Geometry check sheet. Reference: the model listing, model coordinates, mm. A direction names the side the tool comes from. Round coordinates to 2 decimals unless told otherwise and drop trailing zeros. Order: outer loops, then holes, each group sorted by start corner. A loop starts at its lowest first (then second) coordinate and runs counter-clockwise, first axis right, second up. Notation, with made-up numbers: (42.25, 18.5) - (55.25, 18.5) arc R6 ccw to (55.25, 25.5) - close; hole circle Ø10 at (68.5, 79.25). An arc over 180 degrees is marked (long way). One line per question, with ' | ' between items. Start each with the question number.
Q1. Material ranges on line 1 along Y through (x, z) = (11.5, -8); line 2 along Y through (x, z) = (5.25, 5.5); line 3 along X through (y, z) = (18.25, 2.75), recorded low to high.
Q2. Sectioned sample at B-B, the plane z = -6. Enter the section's corners in (x, y).
Q3. Tool access check on faces 1 (the face through (5, 15, 0)), 2 (the face through (17.465, 2.465, -0.14)). Record the directions out of +Z, -Z, +X, -X, +Y, -Y that give a thin tool (end or side, any length) a straight path to the whole face; none if there is none.
Q4. Sectioned sample at C-C, the plane y = 16.5. Enter the section's corners in (x, z).
Q5. Sectioned sample at D-D, the plane z = 0. Enter the section's corners in (x, y), then the cut area to 3 significant figures.
Q6. Gauge pin test, flat ends, axial feed: P1, Ø12, axis at x = 12, z = 3.5, coming from the +Y side; P2, Ø11, axis at x = 4.5, z = 2.5, coming from the +Y side; P3, Ø5, axis at y = 3, z = -3.5, coming from the -X side; P4, Ø4, axis at x = -3.5, y = 3, coming from the +Z side. Record the tip position at first contact, or that the pin passes through.
Q7. Sectioned sample at A-A, the plane x = 7. Enter the section's corners in (y, z), then the cut area to 3 significant figures.
```python
from build123d import *

# Parameters (mm, degrees)
EXTRUDE_2_DEPTH = 20
EXTRUDE_3_DEPTH = 15
EXTRUDE_4_DEPTH = 5


with BuildPart() as part:
    # Sketch 1 → Extrude 2 (new body)
    with BuildSketch(Plane(origin=(0, 0, 0), x_dir=(1, 0, 0), z_dir=(0, 1, 0))):
        with BuildLine():
            Line((5, 10), (0, 10))
            ThreePointArc((0, 10), (-10, 0), (0, -10))
            Line((0, -10), (5, 10))
        make_face()
    extrude(amount=EXTRUDE_2_DEPTH)

    # Sketch 1_4 → Extrude 3 (add)
    with BuildSketch(Plane(origin=(0, 0, 0), x_dir=(1, 0, 0), z_dir=(0, 1, 0))):
        Polygon((10, 10), (5, 10), (0, -10), (5, -10), align=None)
    extrude(amount=EXTRUDE_3_DEPTH)

    # Sketch 1_5 → Extrude 4 (add)
    with BuildSketch(Plane(origin=(0, 0, 0), x_dir=(1, 0, 0), z_dir=(0, 1, 0))):
        with BuildLine():
            Line((0, 10), (15, 10))
            Line((15, 10), (20, -10))
            Line((20, -10), (0, -10))
            ThreePointArc((0, -10), (-10, 0), (0, 10))
        make_face()
    extrude(amount=EXTRUDE_4_DEPTH)


solid = part.part
```
Determined:
1) line 1: y = 0 to 5 | line 2: y = 0 to 15 | line 3: x = -9.61 to 1.81
2) outline: (-8, 0) - (16, 0) - (16, 5) - (9, 5) - (9, 15) - (4, 15) - (4, 20) - (-8, 20) - close
3) face 1: +Z, +X, +Y | face 2: -Z, +X, +Y, -Y
4) outline: (0, -10) - (5, -10) - (0, 10) arc R10 ccw to start
5) outline: (-10, 0) - (17.5, 0) - (17.5, 5) - (7.5, 5) - (7.5, 15) - (2.5, 15) - (2.5, 20) - (-10, 20) - close | area: 375 mm2
6) P1: stops at y = 15 | P2: stops at y = 20 | P3: stops at x = -9.95 | P4: stops at z = 9.89
7) outline: (0, -10) - (15, -10) - (15, 2) - (5, 2) - (5, 10) - (0, 10) - close | area: 220 mm2
